Read the model definition and answer for the solid it produces. Units are mm, in the model's axes. Coordinates: 2 decimals unless noted, no trailing zeros. Loops run counter-clockwise (first coordinate to the right, second up) from the corner with the lowest first, then second, coordinate; pieces in that order, holes last. Notation, with made-up numbers: (46.25, 23) -> (97.25, 23) arc R26 ccw to (97.25, 43) -> close; hole circle Ø7 at (73.5, 63.25). An arc over 180 degrees is marked (long way). Answer as CSV lines item,"result".
```python
from build123d import *

# Parameters (mm, degrees)
BASPROSKE_W        = 12
BASPROSKE_H        = 24
TOOTHCUT_DEPTH     = 37
TEETHCUTS_COUNT    = 10
TEETHCUTS_ANGLE    = 324
HUBNEAONESKE_R     = 8
HUBNEARONE_DEPTH   = 38.0000508
BORSKE_R           = 4
BORE_DEPTH         = 12.0000508
SKETCH1_R          = 10.27069338
CUT_EXTRUDE1_DEPTH = 43


with BuildPart() as part:
    # BasProSke → Base-Revolve (revolve)
    with BuildSketch(Plane(origin=(0, 0, 0), x_dir=(1, 0, 0), z_dir=(0, 1, 0)), mode=Mode.PRIVATE) as base_revolve_sk:
        with Locations((6, 12)):
            Rectangle(BASPROSKE_W, BASPROSKE_H)
    revolve(base_revolve_sk.sketch.rotate(Axis((-10, 0, 0), (1, 0, 0)), 180), axis=Axis((-10, 0, 0), (1, 0, 0)))

    # TooCutSke → ToothCut (cut, through all)
    with BuildSketch(Plane(origin=(0, 0, 0), x_dir=(0, 0, -1), z_dir=(1, 0, 0))):
        with BuildLine():
            ThreePointArc((2.33803632, 14.815653451), (0, 14.999), (-2.33803632, 14.815653451))
            ThreePointArc((-2.33803632, 14.815653451), (-3.315013319, 19.654913653), (-6.946609122, 22.999227528))
            ThreePointArc((-6.946609122, 22.999227528), (0, 24.0254), (6.946609122, 22.999227528))
            ThreePointArc((6.946609122, 22.999227528), (3.315013319, 19.654913653), (2.33803632, 14.815653451))
        make_face()
    toothcut = extrude(amount=TOOTHCUT_DEPTH, mode=Mode.SUBTRACT)

    # TeethCuts: ToothCut ×10 about axis
    teethcuts_axis = Axis((-10, 0, 0), (1, 0, 0))
    for i in range(1, TEETHCUTS_COUNT):
        add(toothcut.rotate(teethcuts_axis, i * TEETHCUTS_ANGLE / (TEETHCUTS_COUNT - 1)), mode=Mode.SUBTRACT)

    # HubNeaOneSke → HubNearOne (add)
    with BuildSketch(Plane.ZY):
        with Locations(Location((0, 0, 0), (0, 0, 180))):
            Circle(HUBNEAONESKE_R)
    extrude(amount=HUBNEARONE_DEPTH)

    # BorSke → Bore (cut, symmetric)
    with BuildSketch(Plane(origin=(0, 0, 0), x_dir=(0, 0, -1), z_dir=(1, 0, 0))):
        with Locations(Location((0, 0, 0), (0, 0, 180))):
            Circle(BORSKE_R)
    extrude(amount=BORE_DEPTH, both=True, mode=Mode.SUBTRACT)

    # Sketch1 → Cut-Extrude1 (cut)
    with BuildSketch(Plane.ZY.offset(10)):
        Circle(SKETCH1_R)
    extrude(amount=CUT_EXTRUDE1_DEPTH, mode=Mode.SUBTRACT)


solid = part.part
```
Q1. For a pull along Z with two mould halves and no side action, classify faces 1 (the face through (1.154, 3.905, -0.867)), 2 (the face through (6, 0, -24)), 3 (the face through (-4.93, 7.81, 1.73)) as pulls with the +Z half, pulls with the -Z half, needs draft (parallel to the pull), parting line crosses it, or undercut.
Results:
face 1,"undercut"
face 2,"pulls with the -Z half"
face 3,"parting line crosses it"
Q2. A cutting plane is placed at D-D, the plane z = 5.5. Write down the section's boundary in (x, y).
Results:
outline,"(-10, -5.81) -> (0, -5.81) -> (0, -22.14) -> (12, -22.14) -> (12, 22.14) -> (0, 22.14) -> (0, 5.81) -> (-10, 5.81) -> close"
Q3. Given pin 1 Ø4 at (x, z) = (9, 11) entering from +Y; pin 2 Ø2 at (x, y) = (8.5, 12.5) entering from -Z; pin 3 Ø2 at (x, y) = (-5.5, 5) entering from +Z; pin 4 Ø10 at (x, z) = (9.5, 9.5) entering from -Y, each flat-ended and moving along its own axis, determine where each tip first touches the part or whether it passes through.
Results:
pin 1,"stops at y = 13.25"
pin 2,"stops at z = -19.7"
pin 3,"stops at z = 6.93"
pin 4,"stops at y = -22.98"
Q4. Find the intervals of material crossed by probe 1 along Y at (x, z) = (5.5, 0); probe 2 along Y at (x, z) = (4, -17); probe 3 along X at (y, z) = (-8, -3), in increasing order. Write a range as [from, to].
Results:
probe 1,"y = [-15, -4], [4, 15]"
probe 2,"y = [-14.66, -8.58], [-3, 3], [8.58, 14.66]"
probe 3,"x = [0, 12]"
Q5. A cutting plane is placed at B-B, the plane y = 19.5. Write down the section's boundary in (x, z).
Results:
outline,"(0, -8.89) -> (12, -8.89) -> (12, -3.23) -> (0, -3.23) -> close; (0, 3.23) -> (12, 3.23) -> (12, 8.89) -> (0, 8.89) -> close"
Q6. A cutting plane is placed at A-A, the plane z = 0. Write down the section's boundary in (x, y).
Results:
outline,"(-10, -8) -> (0, -8) -> (0, -15) -> (12, -15) -> (12, -4) -> (-10, -4) -> close; (-10, 4) -> (12, 4) -> (12, 15) -> (0, 15) -> (0, 8) -> (-10, 8) -> close"
Q7. A cutting plane is placed at C-C, the plane x = -2. Write down the section's boundary in (y, z).
Results:
outline,"circle Ø16 at (0, 0); hole circle Ø8 at (0, 0)"
